```python
from build123d import *

# Parameters (mm, degrees)
SKETCH1_W           = 701.876631599
SKETCH1_H           = 49.976737776
SKETCH1_R           = 5.778560305
BOSS_EXTRUDE1_DEPTH = 3.1


with BuildPart() as part:
    # Sketch1 → Boss-Extrude1 (new body)
    with BuildSketch(Plane(origin=(0, 0, 0), x_dir=(1, 0, 0), z_dir=(0, 1, 0))):
        with Locations((709.588876406, -495.502605974)):
            Rectangle(SKETCH1_W, SKETCH1_H)
        with Locations(Location((383.143601119, -495.502605974, 0), (0, 0, 90))):
            Circle(SKETCH1_R, mode=Mode.SUBTRACT)
        with Locations(Location((433.120338895, -495.502605974, 0), (0, 0, 90))):
            Circle(SKETCH1_R, mode=Mode.SUBTRACT)
        with Locations(Location((483.097076671, -495.502605974, 0), (0, 0, 90))):
            Circle(SKETCH1_R, mode=Mode.SUBTRACT)
        with Locations(Location((533.073814447, -495.502605974, 0), (0, 0, 90))):
            Circle(SKETCH1_R, mode=Mode.SUBTRACT)
        with Locations(Location((583.050552222, -495.502605974, 0), (0, 0, 90))):
            Circle(SKETCH1_R, mode=Mode.SUBTRACT)
        with Locations(Location((633.027289998, -495.502605974, 0), (0, 0, 90))):
            Circle(SKETCH1_R, mode=Mode.SUBTRACT)
        with Locations(Location((683.004027774, -495.502605974, 0), (0, 0, 90))):
            Circle(SKETCH1_R, mode=Mode.SUBTRACT)
        with Locations(Location((732.98076555, -495.502605974, 0), (0, 0, 90))):
            Circle(SKETCH1_R, mode=Mode.SUBTRACT)
        with Locations(Location((782.957503326, -495.502605974, 0), (0, 0, 90))):
            Circle(SKETCH1_R, mode=Mode.SUBTRACT)
        with Locations(Location((832.934241102, -495.502605974, 0), (0, 0, 90))):
            Circle(SKETCH1_R, mode=Mode.SUBTRACT)
        with Locations(Location((882.910978877, -495.502605974, 0), (0, 0, 90))):
            Circle(SKETCH1_R, mode=Mode.SUBTRACT)
        with Locations(Location((932.887716653, -495.502605974, 0), (0, 0, 90))):
            Circle(SKETCH1_R, mode=Mode.SUBTRACT)
        with Locations(Location((982.864454429, -495.502605974, 0), (0, 0, 90))):
            Circle(SKETCH1_R, mode=Mode.SUBTRACT)
        with Locations(Location((1032.841192205, -495.502605974, 0), (0, 0, 90))):
            Circle(SKETCH1_R, mode=Mode.SUBTRACT)
    extrude(amount=BOSS_EXTRUDE1_DEPTH)


solid = part.part
```
CAD build for the part. Positions are in the model's coordinates, mm. Round coordinates to 2 decimals unless told otherwise and drop trailing zeros. Answer as CSV lines item,"result". Start each with the question number.
1. Drill centre lines: L1, parallel to Z at x = 729, y = 0.3; L2, parallel to Z at x = 478.5, y = 2.2. Where is each one in solid material? Low to high. Write a range as [from, to].
2. Pin check, flat tips, straight feed: pin 1 (18.5 mm diameter, centred on x = 433.12, z = 495.5, fed in from -Y); pin 2 (7 mm diameter, centred on x = 633.03, z = 495.5, fed in from +Y). Stop position of each tip, or through.
3. Pull direction Z, two halves, no side cores. Call faces 1 (the face through (705, 3.1, 495)), 2 (the face through (731.25, 1.53, 489.99)), 3 (the face through (1027.11, 1.53, 496.25)): +Z half, -Z half, draft (parallel to the pull), parting line (faces both ways), or undercut.
4. Saw through at A-A, the plane y = 0.75. Count the separate pieces of the cut face and the enclosed holes in it, and give its area (3 significant figures).
Model answer:
1,L1,"z = [470.51, 491.31], [499.69, 520.49]"
1,L2,"z = [470.51, 492], [499, 520.49]"
2,pin 1,"stops at y = 0"
2,pin 2,"passes through"
3,face 1,"draft"
3,face 2,"undercut"
3,face 3,"undercut"
4,separate pieces,"1"
4,enclosed holes,"14"
4,area,"33,600 mm²"
